Part print with two shaded views. Sizes in mm from the minimum x, y, z corner. Give positions to 0.01 mm unless a question says otherwise; leave off trailing zeros. Write each loop counter-clockwise with the first axis right and the second up, starting at its lowest first coordinate (ties: lowest second). Pieces come first, ordered by that corner, then holes. Notation, with made-up numbers: (-6, 12.5) -> (35, 12.5) arc R19 ccw to (35, 35.5) -> close; hole circle Ø2 at (-8, 80.25). An arc over 180 degrees is marked (long way). Write item = value, one per line. Start each with the question number.
Q1. Saw through at A-A, the plane y = 67. List the corners of the cut face in (x, z), then the cut area to 3 significant figures.
Q2. Saw through at C-C, the plane x = 25. List the corners of the cut face in (y, z), then the cut area to 3 significant figures.
Q3. Wall check: line 1 (Y direction, x = 135, z = 151.5); line 2 (X direction, y = 89, z = 19); line 3 (X direction, y = 73.5, z = 9). Give the ranges that are in metal, low to high.
Q4. Saw through at B-B, the plane z = 88. List the corners of the cut face in (x, y), then the cut area to 3 significant figures.
Q5. Mould opens along X. For the marked faces 1 and 2 say: pulls with the +X half, pulls with the -X half, needs draft (parallel to the pull), parting line crosses it, or undercut.
Q6. Drop flat-ended pins along their axis: P1, Ø4, axis at x = 228.5, y = 64, coming from the -Z side; P2, Ø1.4, axis at x = 8, y = 62, coming from the +Z side; P3, Ø16.5, axis at y = 114.5, z = 181.5, coming from the +X side. Give the stop position or say it passes through.
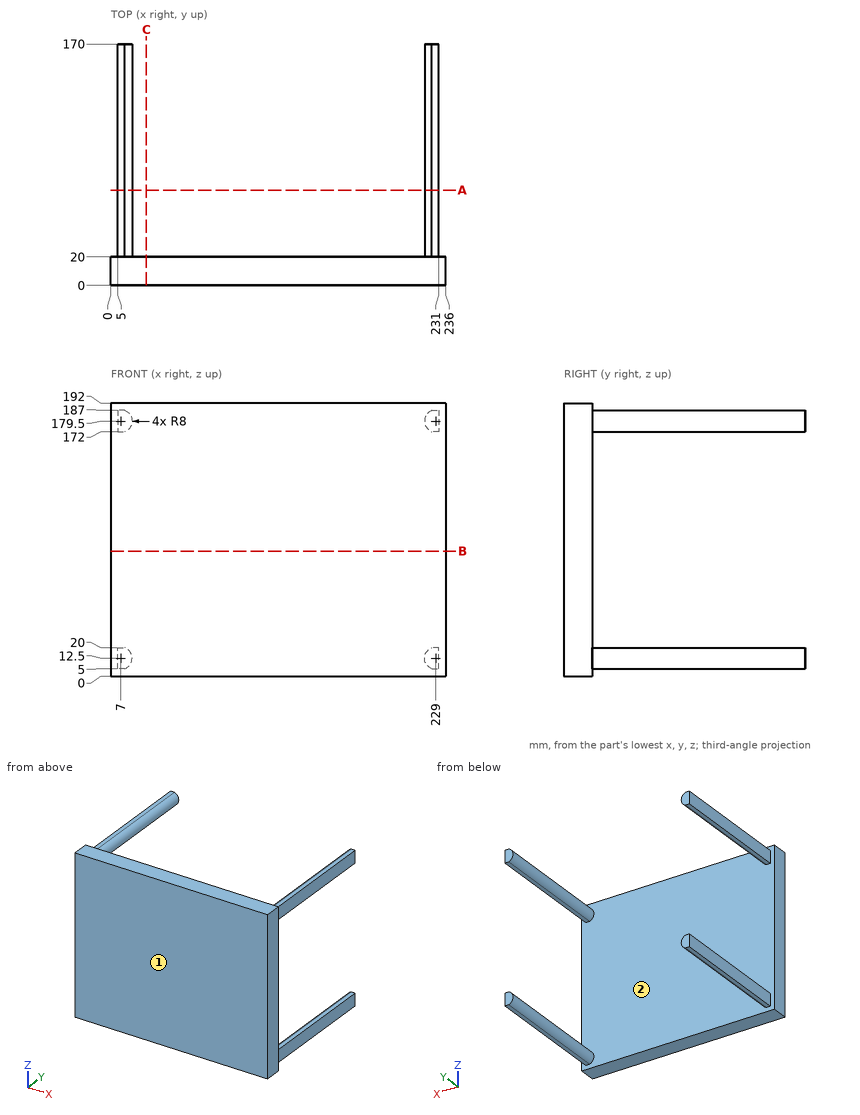
Report:
q1.outline = (5, 5) -> (9.78, 5) arc R8 ccw to (9.78, 20) -> (5, 20) -> close; (5, 172) -> (9.78, 172) arc R8 ccw to (9.78, 187) -> (5, 187) -> close; (226.22, 5) -> (231, 5) -> (231, 20) -> (226.22, 20) arc R8 ccw to start; (226.22, 172) -> (231, 172) -> (231, 187) -> (226.22, 187) arc R8 ccw to start
q1.area = 515 mm2
q2.outline = (0, 0) -> (20, 0) -> (20, 192) -> (0, 192) -> close
q2.area = 3,840 mm2
q3.line_1 = 0 to 20
q3.line_2 = 5 to 11.66, 224.34 to 231
q3.line_3 = 5 to 14.19, 221.81 to 231
q4.outline = (0, 0) -> (236, 0) -> (236, 20) -> (0, 20) -> close
q4.area = 4,720 mm2
q5.face_1 = needs draft
q5.face_2 = undercut
q6.P1 = 5
q6.P2 = 187
q6.P3 = 231
